Geometry check sheet. Reference: the model listing, model coordinates, mm. A direction names the side the tool comes from. Coordinates: 2 decimals unless noted, no trailing zeros. Order: outer loops, then holes, each group sorted by start corner. A loop starts at its lowest first (then second) coordinate and runs counter-clockwise, first axis right, second up. Notation, with made-up numbers: M 64,-35.75 L 101,-35.75 A29 ccw 101,-9.75 Z; hole C 61.25,31.25 d9. An arc over 180 degrees is marked long. One line per item, written item: value. Start each with the question number.
1) Sectioned sample at D-D, the plane x = 124. Enter the section's corners in (y, z).
2) Access from +Z, -Z, +X, -X, +Y, -Y to the whole of each face (thin tool, end or side, straight path). Record for faces 1 (the flat face through (90, -59.436, 42)), 2 (the flat face through (64, -66.04, 59)), 3 (the flat face through (90, 19.05, 40)), 4 (the flat face through (93, 11, 16.51)), 5 (the flat face through (84.08, -64.75, 32.66)).
3) Thickness scan on L1, parallel to X at y = -32, z = 50; L2, parallel to Y at x = 101, z = 39; L3, parallel to Z at x = 114, y = -29. Record the ranges inside material, lowest first. Write a range as from..to.
4) Sectioned sample at B-B, the plane y = 6.5. Enter the section's corners in (x, z).
5) Draft check along Y on faces 6 (the flat face through (87.775, -64.752, 34.267)), 7 (the flat face through (53, -66.04, 48)), 8 (the flat face through (41, -4.064, 4)). Enter one of: pulls with the +Y half, pulls with the -Y half, needs draft (parallel to the pull), parting line crosses it, or undercut.
6) Sectioned sample at A-A, the plane x = 144. Enter the section's corners in (y, z).
7) Go/stop test with flat-tipped pins: P1, Ø6, axis at x = 91, z = 4, coming from the -Y side; P2, Ø6, axis at x = 78.5, y = -54.5, coming from the +Z side; P3, Ø4.5, axis at x = 80, y = -13.5, coming from the +Z side. Record where each tip stops, or that it passes through.
Autodesk Inventor part; units mm, degrees
ref_plane "YZ Plane" through (0, 0, 0) normal (1, 0, 0) x (0, 1, 0)
ref_plane "XZ Plane" through (0, 0, 0) normal (0, 1, 0) x (-1, 0, 0)
ref_plane "XY Plane" through (0, 0, 0) normal (0, 0, 1) x (1, 0, 0)
sketch "Sketch1" plane through (0, 0, 0) normal (0, 0, 1) x (1, 0, 0)
  line L0 (6.35, -116.84) -> (8.89, -119.38)
  line L1 (8.89, -119.38) -> (8.89, -121.92)
  line L2 (6.35, -84.074) -> (6.35, -116.84)
  line L3 (8.89, -81.534) -> (6.35, -84.074)
  line L4 (8.89, -68.58) -> (8.89, -81.534)
  line L5 (74.93, -68.58) -> (8.89, -68.58)
  line L6 (74.93, -121.92) -> (74.93, -68.58)
  line L7 (8.89, -121.92) -> (74.93, -121.92)
  line L8 (5.334, -117.2608) -> (7.874, -119.8008)
  line L9 (7.874, -119.8008) -> (7.874, -122.936)
  line L10 (7.874, -122.936) -> (75.946, -122.936)
  line L11 (75.946, -122.936) -> (75.946, -67.564)
  line L12 (75.946, -67.564) -> (7.874, -67.564)
  line L13 (7.874, -67.564) -> (7.874, -81.1132)
  line L14 (7.874, -81.1132) -> (5.334, -83.6532)
  line L15 (5.334, -83.6532) -> (5.334, -117.2608)
  line L16 (0, -63.5) -> (81.28, -63.5)
  line L17 (81.28, -63.5) -> (81.28, 0)
  line L18 (81.28, 0) -> (0, 0)
  line L19 (0, 0) -> (0, -63.5)
  line L20 (5.334, -111.1172) -> (0, -111.1172) construction
  line L21 (75.946, -101.4463) -> (81.28, -101.4463) construction
  line L22 (34.5139, -122.936) -> (34.5139, -63.5) construction
  line L23 (37.8868, -59.436) -> (37.8868, 0) construction
  line L24 (75.946, -76.28) -> (81.28, -76.28)
  line L25 (75.946, -120.595) -> (81.28, -120.595)
  line L26 (75.946, -107.895) -> (81.28, -107.895)
  line L27 (75.946, -91.52) -> (79.6093, -91.52)
  line L28 (81.28, -89.46) -> (81.28, -78.34)
  line L29 (76.835, -110.245) -> (76.835, -118.245)
  circle A0 centre (8.89, -114.3) radius 1.5875
  circle A1 centre (60.96, -119.38) radius 1.5875
  circle A2 centre (59.69, -71.12) radius 1.5875
  circle A3 centre (8.89, -86.36) radius 1.5875
  circle A4 centre (8.89, -114.3) radius 1.0795
  circle A5 centre (8.89, -86.36) radius 1.0795
  circle A6 centre (59.69, -71.12) radius 1.0795
  circle A7 centre (60.96, -119.38) radius 1.0795
  circle A8 centre (40.64, -95.2527) radius 8.89
  line L30 (6.35, -10.16) -> (8.89, -7.62)
  line L31 (8.89, -7.62) -> (8.89, -5.08)
  line L32 (6.35, -42.926) -> (6.35, -10.16)
  line L33 (8.89, -45.466) -> (6.35, -42.926)
  line L34 (8.89, -58.42) -> (8.89, -45.466)
  line L35 (74.93, -58.42) -> (8.89, -58.42)
  line L36 (74.93, -5.08) -> (74.93, -58.42)
  line L37 (8.89, -5.08) -> (74.93, -5.08)
  line L38 (5.334, -9.7392) -> (7.874, -7.1992)
  line L39 (7.874, -7.1992) -> (7.874, -4.064)
  line L40 (7.874, -4.064) -> (75.946, -4.064)
  line L41 (75.946, -4.064) -> (75.946, -59.436)
  line L42 (75.946, -59.436) -> (7.874, -59.436)
  line L43 (7.874, -59.436) -> (7.874, -45.8868)
  line L44 (7.874, -45.8868) -> (5.334, -43.3468)
  line L45 (5.334, -43.3468) -> (5.334, -9.7392)
  line L46 (5.334, -15.8828) -> (0, -15.8828) construction
  line L47 (75.946, -25.5537) -> (81.28, -25.5537) construction
  line L48 (75.946, -50.72) -> (81.28, -50.72)
  line L49 (75.946, -6.405) -> (81.28, -6.405)
  line L50 (75.946, -19.105) -> (81.28, -19.105)
  line L51 (75.946, -35.48) -> (81.28, -35.48)
  line L52 (81.28, -37.54) -> (81.28, -48.66)
  line L53 (76.835, -16.755) -> (76.835, -8.755)
  circle A9 centre (8.89, -12.7) radius 1.5875
  circle A10 centre (60.96, -7.62) radius 1.5875
  circle A11 centre (59.69, -55.88) radius 1.5875
  circle A12 centre (8.89, -40.64) radius 1.5875
  circle A13 centre (8.89, -12.7) radius 1.0795
  circle A14 centre (8.89, -40.64) radius 1.0795
  circle A15 centre (59.69, -55.88) radius 1.0795
  circle A16 centre (60.96, -7.62) radius 1.0795
  circle A17 centre (40.64, -31.7473) radius 8.89
  point P0 (0, 0)
  point P1 (81.28, -130.1977)
  point P2 (77.7776, -91.52)
  point P3 (81.28, -83.9)
  point P4 (76.835, -114.245)
  point P5 (8.89, -120.65)
  point P6 (41.91, -121.92)
  point P7 (81.28, 3.1977)
  point P8 (34.5139, -4.064)
  point P9 (79.6093, -35.48)
  point P10 (77.7776, -35.48)
  point P11 (81.28, -43.1)
  point P12 (76.835, -12.755)
  point P13 (8.89, -6.35)
  point P14 (41.91, -5.08)
  dimension "d0" = 1.016
  dimension "d1" = 81.28
  dimension "d2" = 63.5
  dimension "d3" = 15.24
  dimension "d4" = 7.62
  dimension "d5" = 12.7
  dimension "d6" = 6.35
  dimension "d7" = 2.159
  dimension "d8" = 2.159
  dimension "d9" = 2.159
  dimension "d10" = 2.159
  dimension "d38" = 17.78
  dimension "d40" = 40.64
  dimension "d93" = 5.334
  dimension "d94" = 63.5
  dimension "d96" = 55.372
  dimension "d97" = 4.064
  dimension "d98" = 4.6592
  dimension "d99" = 2.54
  dimension "d100" = 12.954
  dimension "d101" = 12.5332
  dimension "d102" = 15.0732
  dimension "d103" = 15.494
  dimension "d104" = 6.35
  dimension "d105" = 35.56
  dimension "d106" = 2.54
  dimension "d107" = 50.8
  dimension "d108" = 6.1261
  dimension "d109" = 1.27
  dimension "d110" = 26.6673
extrude "Extrusion1" add sketch "Sketch1" against normal blind 2.54 contours L19 L18 L17 L49 L41 L40 L39 L38 L45 L44 L43 L42 L48 L16 | L48 L41 L51 L17 | L41 L42 L43 L44 L45 L38 L39 L40 | L17 L50 L41 L49 | L41 L50 L17 L51 | L30 L31 L37 L36 L35 L34 L33 L32 | A9 | A10 | A11 | A12 | A13 | A14 | A15 | A16 | A17
extrude "Extrusion2" add sketch "Sketch1" along normal blind 7.62 contours L19 L18 L17 L49 L41 L40 L39 L38 L45 L44 L43 L42 L48 L16 | L41 L50 L17 L51 | A9 | A10 | A11 | A12 | A13 | A14 | A15 | A16
extrude "Extrusion4" add sketch "Sketch1" along normal blind 2.54 contours L19 L18 L17 L49 L41 L40 L39 L38 L45 L44 L43 L42 L48 L16 | L48 L41 L51 L17 | L17 L50 L41 L49 | L41 L50 L17 L51 | A9 | A10 | A11 | A12 | A13 | A14 | A15 | A16
sketch "Sketch9" plane through (0, 0, -2.54) normal (0, 0, -1) x (-1, 0, 0)
  line L0 (-81.28, -6.405) -> (-81.28, 0)
  line L1 (0, 0) -> (-81.28, 0)
  line L2 (-81.28, -63.5) -> (0, -63.5)
  line L3 (-81.28, 0) -> (-81.28, -63.5)
  line L4 (-81.28, -63.5) -> (-182.88, -63.5)
  line L5 (-182.88, -63.5) -> (-182.88, 19.05)
  line L6 (-182.88, 19.05) -> (0, 19.05)
  line L7 (0, 19.05) -> (0, 0)
  dimension "d115" = 182.88
  dimension "d116" = 19.05
extrude "Extrusion14" add sketch "Sketch9" against normal up to surface (10.16 mm away)
sketch "Sketch10" plane through (0, 0, 7.62) normal (0, 0, 1) x (1, 0, 0)
  line L0 (81.28, -19.105) -> (81.28, -6.405)
  line L1 (81.28, -50.72) -> (81.28, -35.48)
  line L2 (0, -63.5) -> (182.88, -63.5)
  line L3 (81.28, -6.405) -> (157.48, -6.405)
  line L4 (157.48, -6.405) -> (157.48, -63.5)
  line L5 (157.48, -63.5) -> (81.28, -63.5)
  line L6 (81.28, -63.5) -> (81.28, -6.405)
  point P0 (0, 0)
  dimension "d119" = 76.2
extrude "Extrusion15" cut sketch "Sketch10" against normal up to surface (7.62 mm away)
fillet "Fillet1" radius 38.1 1 edges at (157.48, -6.405, 3.81)
sketch "Sketch11" plane through (0, 19.05, -2.54) normal (0, 1, 0) x (1, 0, 0)
  line L0 (0, 0) -> (0, -10.16)
  line L1 (0, 0) -> (182.88, 0)
  line L2 (182.88, 0) -> (182.88, -86.36)
  line L3 (182.88, -86.36) -> (0, -86.36)
  line L4 (0, -86.36) -> (0, 0)
  line L5 (182.88, 0) -> (182.88, -10.16)
  line L6 (0, -10.16) -> (182.88, -10.16)
  point P0 (0, -2.54)
  dimension "d123" = 76.2
extrude "Extrusion16" add sketch "Sketch11" against normal blind 10.16 contours L6 L2 L3 L4
sketch "Sketch12" plane through (0, 8.89, -2.54) normal (0, -1, 0) x (1, 0, 0)
  line L0 (6.985, 77.47) -> (175.895, 77.47)
  line L1 (175.895, 77.47) -> (175.895, 19.05)
  line L2 (175.895, 19.05) -> (6.985, 19.05)
  line L3 (6.985, 19.05) -> (6.985, 77.47)
  line L4 (0, 86.36) -> (0, 10.16)
  line L5 (182.88, 86.36) -> (0, 86.36)
  point P0 (0, 2.54)
  point P1 (91.44, 77.47)
  point P2 (91.44, 86.36)
  point P3 (6.985, 48.26)
  point P4 (0, 48.26)
  dimension "d126" = 168.91
  dimension "d127" = 58.42
extrude "Extrusion17" cut sketch "Sketch12" against normal blind 5.08
sketch "Sketch13" plane through (0, 0, 7.62) normal (0, 0, 1) x (1, 0, 0)
  line L0 (182.88, 8.89) -> (0, 8.89)
  line L1 (5.334, 8.89) -> (5.334, -59.436)
  line L2 (5.334, -59.436) -> (177.546, -59.436)
  line L3 (177.546, -59.436) -> (177.546, 8.89)
  line L4 (182.88, 8.89) -> (182.88, -63.5)
  line L5 (0, -63.5) -> (0, 8.89)
  line L6 (0, -63.5) -> (81.28, -63.5)
  line L7 (157.48, -63.5) -> (81.28, -63.5)
  line L8 (157.48, -63.5) -> (182.88, -63.5)
  point P0 (0, 0)
  point P1 (7.874, -59.436)
  point P2 (5.334, -43.3468)
  point P3 (177.546, -25.273)
  dimension "d131" = 5.334
extrude "Extrusion18" add sketch "Sketch13" along normal up to surface (76.2 mm away) contours L4 L8 L7 L6 L5 L0 L1 L2 L3
sketch "Sketch14" plane through (0, -63.5, -2.54) normal (0, -1, 0) x (1, 0, 0)
  line L0 (81.28, 10.16) -> (157.48, 10.16)
  line L1 (81.28, 5.08) -> (81.28, 10.16)
  line L2 (81.28, 10.16) -> (157.48, 10.16)
  line L3 (157.48, 10.16) -> (157.48, 21.59)
  line L4 (157.48, 21.59) -> (81.28, 21.59)
  line L5 (81.28, 21.59) -> (81.28, 10.16)
  line L6 (157.48, 2.54) -> (81.28, 2.54)
  point P0 (0, 2.54)
  dimension "d134" = 19.05
extrude "Extrusion19" cut sketch "Sketch14" against normal blind 20.6375
sketch "Sketch15" plane through (0, -63.5, -2.54) normal (0, -1, 0) x (1, 0, 0)
  line L0 (81.28, 21.59) -> (81.28, 10.16)
  line L1 (157.48, 2.54) -> (119.38, 2.54)
  line L2 (81.28, 21.59) -> (132.08, 21.59)
  line L3 (132.08, 21.59) -> (132.08, 2.54)
  line L4 (132.08, 2.54) -> (81.28, 2.54)
  line L5 (81.28, 2.54) -> (81.28, 21.59)
  line L6 (157.48, 21.59) -> (157.48, 2.54)
  point P0 (0, 2.54)
  dimension "d137" = 25.4
extrude "Extrusion20" add sketch "Sketch15" against normal up to surface (4.064 mm away)
sketch "Sketch16" plane through (0, -63.5, -2.54) normal (0, -1, 0) x (1, 0, 0)
  line L0 (82.6763, 9.3083) -> (61.6198, 9.2379)
  line L1 (61.6198, 9.2379) -> (51.0306, 27.4381)
  line L2 (51.0306, 27.4381) -> (61.4978, 45.7088)
  line L3 (61.4978, 45.7088) -> (82.5543, 45.7792)
  line L4 (82.5543, 45.7792) -> (93.1436, 27.579)
  line L5 (93.1436, 27.579) -> (82.6763, 9.3083)
  line L6 (64.5477, 40.4668) -> (57.0952, 27.4584)
  line L7 (57.0952, 27.4584) -> (64.6346, 14.5002)
  line L8 (64.6346, 14.5002) -> (79.6264, 14.5503)
  line L9 (79.6264, 14.5503) -> (87.0789, 27.5587)
  line L10 (87.0789, 27.5587) -> (79.5395, 40.5169)
  line L11 (79.5395, 40.5169) -> (64.5477, 40.4668)
  line L12 (51.0044, 35.8885) -> (50.9339, 56.9531)
  line L13 (50.9339, 56.9531) -> (56.2001, 56.9707)
  line L14 (56.2001, 56.9707) -> (56.24, 45.0273)
  line L15 (56.24, 45.0273) -> (51.0044, 35.8885)
  line L16 (61.4193, 71.0002) -> (66.6855, 71.0179)
  line L17 (66.6855, 71.0179) -> (66.7559, 49.9533)
  line L18 (82.5544, 50.0062) -> (82.4839, 71.0707)
  line L19 (82.4839, 71.0707) -> (77.2177, 71.0531)
  line L20 (77.2177, 71.0531) -> (77.2882, 49.9885)
  line L21 (93.1336, 35.9943) -> (93.063, 57.094)
  line L22 (93.063, 57.094) -> (87.7969, 57.0764)
  line L23 (87.7969, 57.0764) -> (87.837, 45.0979)
  line L24 (87.837, 45.0979) -> (93.1336, 35.9943)
  line L25 (69.3009, 76.2928) -> (69.389, 49.9621)
  line L26 (69.389, 49.9621) -> (74.6552, 49.9797)
  line L27 (74.6552, 49.9797) -> (74.5671, 76.3104)
  line L28 (74.5671, 76.3104) -> (69.3009, 76.2928)
  line L29 (77.2882, 49.9885) -> (82.5544, 50.0062)
  line L30 (66.6855, 71.0179) -> (69.3185, 71.0267) construction
  line L31 (77.2177, 71.0531) -> (74.5847, 71.0443) construction
  line L32 (61.4193, 71.0002) -> (61.4898, 49.9357)
  line L33 (61.4898, 49.9357) -> (66.7559, 49.9533)
  point P0 (0, 2.54)
  point P1 (72.0871, 27.5085)
  point P2 (95.9605, 86.1193)
  dimension "d140" = 21.0566
  dimension "d141" = 5.2522
  dimension "d142" = 4.2234
  dimension "d143" = 4.2234
  dimension "d144" = 5.2662
  dimension "d145" = 5.2662
  dimension "d146" = 5.2662
  dimension "d147" = 5.2662
  dimension "d148" = 4.2269
  dimension "d149" = 21.0647
  dimension "d150" = 21.0647
  dimension "d151" = 26.3309
  dimension "d152" = 5.2662
  dimension "d153" = 5.2662
  dimension "d154" = 5.2662
  dimension "d155" = 2.6331
  dimension "d156" = 5.2578
extrude "Extrusion21" add sketch "Sketch16" along normal blind 2.54
chamfer "Chamfer3" distance 2.54 angle 45 11 edges at (90.4853, -66.04, 38.0061) (79.9213, -66.04, 47.4573) (72.0221, -66.04, 47.4309) (64.1229, -66.04, 47.4045) (53.6222, -66.04, 37.9179) (56.3252, -66.04, 15.798) (72.1481, -66.04, 6.7331) (87.9099, -66.04, 15.9036) (83.3092, -66.04, 31.4978) (72.0436, -66.04, 37.9518) (60.8215, -66.04, 31.4226)
equation "\"d8\" = d7"
equation "\"d9\" = d7"
equation "\"d10\" = d7"
properties part number "Liv Mas Base Box"
Final values:
1. outline: M -63.5,-2.54 L 19.05,-2.54 L 19.05,83.82 L 8.89,83.82 L 8.89,74.93 L 13.97,74.93 L 13.97,16.51 L 8.89,16.51 L 8.89,7.62 L -6.69,7.62 L -6.69,0 L -59.44,0 L -59.44,83.82 L -63.5,83.82 Z
2. face 1: +Z
2. face 2: +Z, -Z, +X, -X, -Y
2. face 3: +Z, -Z, +X, -X, +Y
2. face 4: none
2. face 5: -Y
3. L1: x = 0..5.33, 177.55..182.88
3. L2: y = -63.5..-59.44, 13.97..19.05
3. L3: z = -2.54..0
4. outline: M 0,-2.54 L 182.88,-2.54 L 182.88,83.82 L 177.55,83.82 L 177.55,7.62 L 5.33,7.62 L 5.33,83.82 L 0,83.82 Z
5. face 6: needs draft
5. face 7: pulls with the -Y half
5. face 8: undercut
6. outline: M -63.5,-2.54 L 19.05,-2.54 L 19.05,83.82 L 8.89,83.82 L 8.89,74.93 L 13.97,74.93 L 13.97,16.51 L 8.89,16.51 L 8.89,7.62 L -15.43,7.62 L -15.43,0 L -63.5,0 Z; M -63.5,19.05 L -59.44,19.05 L -59.44,83.82 L -63.5,83.82 Z
7. P1: stops at y = -63.5
7. P2: stops at z = 7.62
7. P3: stops at z = 2.54
